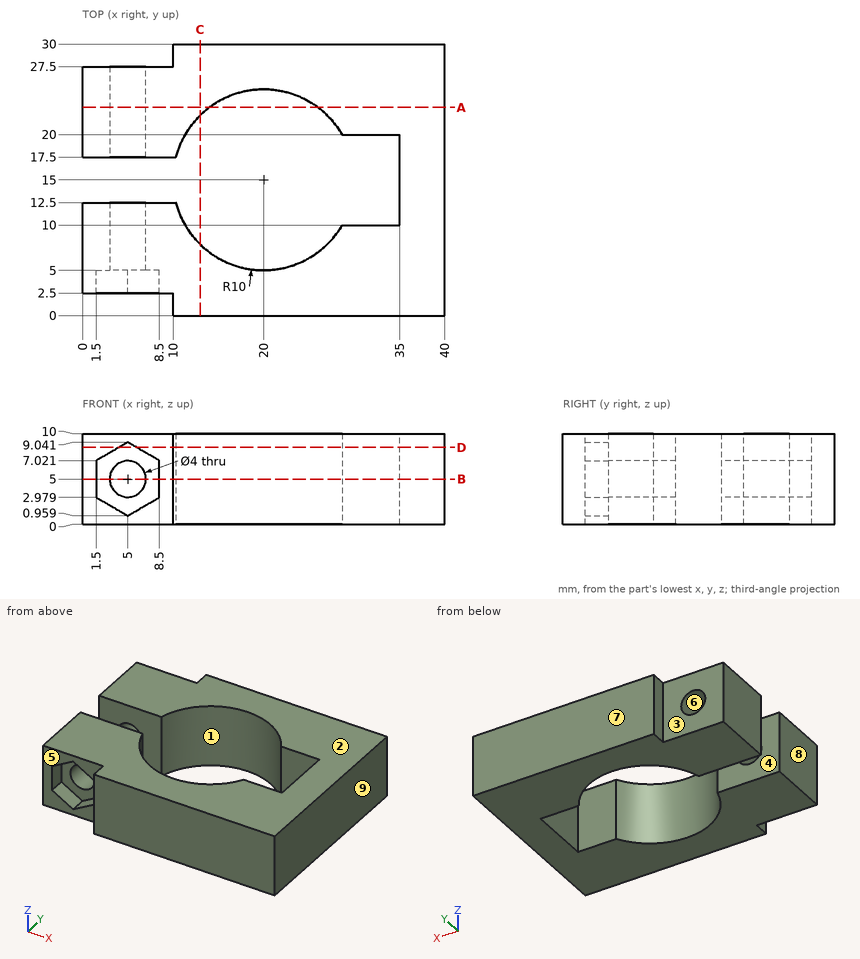
Drawing for the job (mm, zero at the part's lowest x, y, z). A direction names the side the tool comes from. Give positions to 0.01 mm unless a question says otherwise; leave off trailing zeros. Loops run counter-clockwise (first coordinate to the right, second up) from the corner with the lowest first, then second, coordinate; pieces in that order, holes last. Notation, with made-up numbers: M 15.25,11 L 41.25,11 A4 cw 41.25,16 Z; hole C 45,88 d6. An arc over 180 degrees is marked long. Use one line per item in the form item = value.
Item 1: Drill centre lines: probe 1 along Y at (x, z) = (30, 9.75); probe 2 along Z at (x, y) = (5, 23.25); probe 3 along Y at (x, z) = (20, 1.5). Where is each one in solid material? Low to high. Write a range as from..to.
Determined:
probe_1 = 0..10, 20..30
probe_2 = 0..3, 7..10
probe_3 = 0..5, 25..30
Item 2: Which spindle directions (+Z, -Z, +X, -X, +Y, -Y) get a long thin tool onto all of the face, cutting with end or side? Do the marked faces 1, 2, 3, 4 and 5. Say none if no direction does.
Determined:
face_1 = +Z, -Z
face_2 = +Z, +X, -X, +Y, -Y
face_3 = +Z, -Z, -X, +Y
face_4 = +Z, -Z, -X
face_5 = +Z, -Z, -X, -Y
Item 3: Slice it at C-C (x = 13). List the corners of the cut face in (y, z).
Determined:
outline = M 0,0 L 7.86,0 L 7.86,10 L 0,10 Z; M 22.14,0 L 30,0 L 30,10 L 22.14,10 Z
Item 4: Slice it at B-B (z = 5). List the corners of the cut face in (x, y).
Determined:
outline = M 0,2.5 L 1.5,2.5 L 1.5,5 L 3,5 L 3,12.5 L 0,12.5 Z; M 0,17.5 L 3,17.5 L 3,27.5 L 0,27.5 Z; M 7,5 L 8.5,5 L 8.5,2.5 L 10,2.5 L 10,0 L 40,0 L 40,30 L 10,30 L 10,27.5 L 7,27.5 L 7,17.5 L 10.32,17.5 A10 cw 28.66,20 L 35,20 L 35,10 L 28.66,10 A10 cw 10.32,12.5 L 7,12.5 Z
Item 5: Slice it at A-A (y = 23). List the corners of the cut face in (x, z).
Determined:
outline = M 0,0 L 14,0 L 14,10 L 0,10 Z; M 26,0 L 40,0 L 40,10 L 26,10 Z; hole C 5,5 d4
Item 6: Slice it at D-D (z = 8.5). List the corners of the cut face in (x, y).
Determined:
outline = M 0,2.5 L 4.06,2.5 L 4.06,5 L 5.94,5 L 5.94,2.5 L 10,2.5 L 10,0 L 40,0 L 40,30 L 10,30 L 10,27.5 L 0,27.5 L 0,17.5 L 10.32,17.5 A10 cw 28.66,20 L 35,20 L 35,10 L 28.66,10 A10 cw 10.32,12.5 L 0,12.5 Z
Item 7: Two-plate mould, pull along X, no slides. Class the marked faces 6, 7, 8 and 9: pulls with the +X half, pulls with the -X half, needs draft (parallel to the pull), parting line crosses it, or undercut.
Determined:
face_6 = undercut
face_7 = needs draft
face_8 = pulls with the -X half
face_9 = pulls with the +X half
Item 8: Flat gauge pins, fed straight in: pin 1 (5 mm diameter, centred on x = 5.5, z = 4.5, fed in from -Y); pin 2 (0.8 mm diameter, centred on y = 1, z = 3, fed in from -X); pin 3 (5 mm diameter, centred on x = 6.5, z = 5.5, fed in from +Y). Where does each tip first touch, or does it go through?
Determined:
pin_1 = 5
pin_2 = 10
pin_3 = 27.5
